```python
from build123d import *

# Parameters (mm, degrees)
F1_DEPTH  = 30
F2_W      = 12
F2_H      = 7
F3_DEPTH  = 38.2116781187
F5_DEPTH  = 25
F6_W      = 60.886583291
F6_H      = 11.9508793578
F7_DEPTH  = 25
F8_W      = 14
F8_H      = 9
F8_W_2    = 11
F8_H_2    = 6
F9_DEPTH  = 3.5
F10_W     = 41.5411135182
F10_H     = 24.3398016319
F11_DEPTH = 25


with BuildPart() as f1:
    # F0 (on Front) → F1 (new body, symmetric)
    with BuildSketch(Plane.XZ):
        Polygon((-8.4852813742, 41.5147186258), (-35.8526408672, 14.1473591328), (-35.8526408672, 0), (50, 0), (21.2132034356, 28.7867965644), (12.7279220614, 20.3015151902), align=None)
    extrude(amount=F1_DEPTH, both=True)

    # F2 (on face) → F3 (cut, through all)
    with BuildSketch(Plane(origin=(-3.7867965644, 0, 3.7867965644), x_dir=(0, -1, 0), z_dir=(-0.7071067812, 0, 0.7071067812))):
        with Locations((0, 29.3553390593)):
            Rectangle(F2_W, F2_H)
    extrude(amount=-F3_DEPTH, mode=Mode.SUBTRACT)

    # F4 (on Front) → F5 (cut, symmetric)
    with BuildSketch(Plane.XZ):
        with BuildLine():
            Line((31.8941702423, 0), (46.1681298912, 0))
            Line((46.1681298912, 0), (26.9125392085, 19.3730033934))
            ThreePointArc((26.9125392085, 19.3730033934), (19.7053909545, 19.0432368727), (12.7481166376, 17.1332457749))
            Line((12.7481166376, 17.1332457749), (12.7279220614, 6.3964259197))
            ThreePointArc((12.7279220614, 6.3964259197), (17.3138400367, 8.572904137), (22.2663749009, 9.6865016967))
            Line((22.2663749009, 9.6865016967), (31.8941702423, 0))
        make_face()
    extrude(amount=F5_DEPTH, both=True, mode=Mode.SUBTRACT)

    # F6 (on Front) → F7 (cut, symmetric)
    with BuildSketch(Plane.XZ):
        with Locations((-8.9317080565, 5.9754396789)):
            Rectangle(F6_W, F6_H)
    extrude(amount=F7_DEPTH, both=True, mode=Mode.SUBTRACT)

    # F8 (on face) → F9 (join, symmetric)
    with BuildSketch(Plane(origin=(-3.7867965644, 0, 3.7867965644), x_dir=(0, -1, 0), z_dir=(-0.7071067812, 0, 0.7071067812))):
        with Locations((0, 29.3553390593)):
            Rectangle(F8_W, F8_H)
        with Locations((0, 29.3553390593)):
            Rectangle(F8_W_2, F8_H_2, mode=Mode.SUBTRACT)
    extrude(amount=F9_DEPTH, both=True)

    # F10 (on Front) → F11 (cut, symmetric)
    with BuildSketch(Plane.XZ):
        with Locations((-29.2559308, 29.3487575836)):
            Rectangle(F10_W, F10_H)
    extrude(amount=F11_DEPTH, both=True, mode=Mode.SUBTRACT)


solid = f1.part
```
For this review, take the finished solid that the model builds, in its own axes (mm). A direction names the side the tool comes from. Give positions to 0.01 mm unless a question says otherwise; leave off trailing zeros. Loops run counter-clockwise (first coordinate to the right, second up) from the corner with the lowest first, then second, coordinate; pieces in that order, holes last. Notation, with made-up numbers: M 57.25,14 L 93.25,14 A29 cw 93.25,37 Z; hole C 29.5,-38 d9. An arc over 180 degrees is marked long. One line per item, written item: value. Start each with the question number.
Q1. For L1, parallel to Y at x = 0, z = 9; L2, parallel to X at y = -1.5, z = 24; L3, parallel to Y at x = 14, z = 25, list the stretches that pass through material, from the lowest coordinate up.
Q2. Add section C-C (y = -1). Count the separate pieces of the cut face and the enclosed holes in it, and give its area (3 significant figures).
Q3. Machinability: for faces 1 (the face through (25, 6, 20)), 2 (the face through (21.512, 0, 5)), 3 (the face through (18.9, 0.1, 28.98)), which of the approach directions +Z, -Z, +X, -X, +Y, -Y give a long, thin tool a straight path to every point of the face, cutting with its end or side? Answer none if there is none.
Q4. Draft analysis for pull direction Y (two halves, no side actions). For faces 4 (the face through (34.021, 0.084, 12.444)), 5 (the face through (13.259, -0.42, 20.832)), state which applies: released by +Y, released by -Y, zero draft, split by the parting line, or undercut.
Q5. Add section B-B (x = -26). Give the boundary of the cut face in (y, z).
Q6. Clearance check with flat-ended pins moving along their axes: pin 1 Ø1.5 at (x, y) = (10.5, 17) entering from -Z; pin 2 Ø7.5 at (y, z) = (-5.5, 5) entering from -X; pin 3 Ø5 at (x, y) = (-8.5, -14) entering from +Z. State where each tip first meets the part, or that it passes through.
Q7. Add section D-D (x = 26). Give the boundary of the cut face in (y, z).
Reply:
1. L1: -30 to -25, 25 to 30
1. L2: -8.49 to 9.03, 11.48 to 13.27, 22.46 to 26
1. L3: -7 to -5.5, 5.5 to 7
2. separate pieces: 3
2. enclosed holes: 0
2. area: 721 mm²
3. face 1: none
3. face 2: -Z, -X
3. face 3: +Z, +Y, -Y
4. face 4: undercut
4. face 5: zero draft
5. outline: M -30,0 L -25,0 L -25,11.95 L 25,11.95 L 25,0 L 30,0 L 30,24 L 25,24 L 25,17.18 L -25,17.18 L -25,24 L -30,24 Z
6. pin 1: z = 11.95
6. pin 2: x = 21.51
6. pin 3: z = 41.51
7. outline: M -30,0 L 30,0 L 30,24 L -30,24 Z; hole M -25,5.93 L 25,5.93 L 25,19.42 L 6,19.42 L 6,20.46 L -6,20.46 L -6,19.42 L -25,19.42 Z
